Autodesk Inventor part; units mm, degrees
ref_plane "YZ Plane" through (0, 0, 0) normal (1, 0, 0) x (0, 1, 0)
ref_plane "XZ Plane" through (0, 0, 0) normal (0, 1, 0) x (-1, 0, 0)
ref_plane "XY Plane" through (0, 0, 0) normal (0, 0, 1) x (1, 0, 0)
sketch "Sketch1" plane through (0, 0, 0) normal (0, 1, 0) x (-1, 0, 0)
  circle A0 centre (0, 0) radius 5
  line L0 (0, 0) -> (12.5, 0)
  line L1 (12.5, 10) -> (12.5, -10) construction
  line L2 (11, 10) -> (11, -10)
  line L3 (14, -10) -> (14, 10)
  arc A1 (14, 10) -> (11, 10) centre (12.5, 10) ccw
  arc A2 (11, -10) -> (14, -10) centre (12.5, -10) ccw
  circle A3 centre (0, 0) radius 24
  line L4 (0, 0) -> (-33.5, 0)
  line L5 (0, 0) -> (0, 43.5)
  line L6 (-33.5, 0) -> (-33.5, 40)
  line L7 (-33.5, 40) -> (26.5, 40)
  line L8 (26.5, 40) -> (26.5, -35)
  line L9 (26.5, -35) -> (-33.5, -35)
  line L10 (-33.5, -35) -> (-33.5, 0)
  line L11 (-33.5, 40) -> (-13.5, 40)
  line L12 (-13.5, 40) -> (6.5, 40)
  line L13 (6.5, 40) -> (6.5, 45)
  line L14 (6.5, 45) -> (-13.5, 45)
  line L15 (-13.5, 45) -> (-13.5, 40)
  line L16 (-33.5, 40) -> (-33.5, 15)
  line L17 (-33.5, 15) -> (-38.5, 15)
  line L18 (-38.5, 15) -> (-38.5, -5.425)
  line L19 (-38.5, -5.425) -> (-33.5, -5.425)
  line L20 (-33.5, -5.425) -> (-33.5, 15)
  line L21 (-33.5, 15) -> (-35, 15)
  line L22 (-35, 15) -> (-35, 10)
  line L23 (-35, 10) -> (-36.5, 10)
  line L24 (-36.5, 10) -> (-36.5, 0)
  line L25 (-36.5, 0) -> (-35, 0)
  line L26 (-35, 0) -> (-35, 10)
  line L27 (6.5, 40) -> (1.5, 40)
  line L28 (1.5, 40) -> (1.5, 41.5)
  line L29 (1.5, 41.5) -> (-8.5, 41.5)
  line L30 (-8.5, 41.5) -> (-8.5, 43)
  line L31 (-8.5, 43) -> (1.5, 43)
  line L32 (1.5, 43) -> (1.5, 41.5)
  line L33 (0, 0) -> (23.3345, -23.3345)
  line L34 (0, 0) -> (33, 0) construction
  circle A4 centre (23.3345, -23.3345) radius 1.5
  circle A5 centre (23.3345, 23.3345) radius 1.5
  circle A6 centre (-23.3345, 23.3345) radius 1.5
  circle A7 centre (-23.3345, -23.3345) radius 1.5
  line L35 (-11, 10) -> (-11, -10)
  line L36 (-14, -10) -> (-14, 10)
  arc A8 (-11, 10) -> (-14, 10) centre (-12.5, 10) ccw
  arc A9 (-14, -10) -> (-11, -10) centre (-12.5, -10) ccw
  point P0 (6.5, 40)
  dimension "d0" = 10
  dimension "d1" = 12.5
  dimension "d2" = 10
  dimension "d3" = 3
  dimension "d6" = 48
  dimension "d7" = 33.5
  dimension "d8" = 43.5
  dimension "d9" = 60
  dimension "d10" = 75
  dimension "d11" = 20
  dimension "d12" = 20
  dimension "d13" = 5
  dimension "d14" = 25
  dimension "d15" = 5
  dimension "d16" = 1.5
  dimension "d17" = 5
  dimension "d18" = 1.5
  dimension "d19" = 10
  dimension "d20" = 5
  dimension "d21" = 1.5
  dimension "d22" = 10
  dimension "d23" = 1.5
  dimension "d24" = 33
  dimension "d25" = 45
  dimension "d26" = 3
  dimension "d29" = 360
extrude "Extrusion1" add sketch "Sketch1" along normal blind 2 contours A0 L5 A3 L33 | A0 L4 L35 A8 L36 A3 L5 | L33 A3 L4 L36 A9 L35 A0 | L5 L7 L8 L9 L10 L4 A3 | A3 L4 L6 L7 L5 | L7 L15 L14 L13 L28 L32 L31 L30 L29 L5 | L5 L29 L28 L7 | L26 L25 L24 L23 | L10 L19 L18 L17 L6
extrude "Extrusion2" cut sketch "Sketch1" along normal blind 2 contours L26 L25 L24 L23
sketch "Sketch2" plane through (0, 2, 0) normal (0, 1, 0) x (1, 0, 0)
  line L0 (0, -7) -> (0, 7) construction
  line L1 (5, -7) -> (5, 7)
  line L2 (-5, 7) -> (-5, -7)
  arc A0 (-5, -7) -> (5, -7) centre (0, -7) ccw
  arc A1 (5, 7) -> (-5, 7) centre (0, 7) ccw
  point P0 (0, 0)
  dimension "d35" = 7
  dimension "d36" = 10
extrude "Extrusion3" cut sketch "Sketch2" against normal blind 10
properties part number "mount"
Model file for the job. Use its own axes, mm. A direction names the side the tool comes from. Give positions to 0.01 mm unless a question says otherwise; leave off trailing zeros. Order: outer loops, then holes, each group sorted by start corner. A loop starts at its lowest first (then second) coordinate and runs counter-clockwise, first axis right, second up. Notation, with made-up numbers: (69, -34) -> (128, -34) arc R15 cw to (128, -11) -> close; hole circle Ø10 at (73, 62). An arc over 180 degrees is marked (long way). Use CSV: the item, a comma, the result in double quotes.
1. Drill centre lines: line 1 along X through (y, z) = (1.45, -7); line 2 along X through (y, z) = (1.6, 7); line 3 along Z through (x, y) = (6.5, 1.95). Where is each one in solid material? Low to high. Write a range as from..to.
Outcome:
line 1,"-26.5..-14, -11..-5, 5..11, 14..33.5"
line 2,"-26.5..-14, -11..-5, 5..11, 14..35, 36.5..38.5"
line 3,"-35..41.5, 43..45"
2. Band-saw the part on A-A, the plane z = 3. Give the cut face in (x, y), then the cut area to 3 significant figures.
Outcome:
outline,"(-26.5, 0) -> (-14, 0) -> (-14, 2) -> (-26.5, 2) -> close; (-11, 0) -> (-5, 0) -> (-5, 2) -> (-11, 2) -> close; (5, 0) -> (11, 0) -> (11, 2) -> (5, 2) -> close; (14, 0) -> (35, 0) -> (35, 2) -> (14, 2) -> close; (36.5, 0) -> (38.5, 0) -> (38.5, 2) -> (36.5, 2) -> close"
area,"95.0 mm²"
3. 3-axis set-ups, long thin cutter, end or side, ignore diameter. For faces 5 (the flat face through (-6.5, 1, 42)), 6 (the flat face through (4, 1, 43)), 7 (the flat face through (13.5, 1, 43)), 8 (the flat face through (36, 1, -5.425)): which of +Z, -Z, +X, -X, +Y, -Y reach the whole face in a straight line?
Outcome:
face 5,"+Z, -X, +Y, -Y"
face 6,"+Y, -Y"
face 7,"+Z, +X, +Y, -Y"
face 8,"-Z, +X, +Y, -Y"
4. Band-saw the part on D-D, the plane y = 1.6. Count the separate pieces of the cut face and the enclosed holes in it, then the cut area to 3 significant figures.
Outcome:
separate pieces,"1"
enclosed holes,"9"
area,"4,290 mm²"
5. Drop flat-ended pins along their axis: pin 1 (1.2 mm diameter, centred on y = 1.5, z = 42, fed in from -X); pin 2 (2.5 mm diameter, centred on x = 23.33, z = -23.33, fed in from +Y); pin 3 (1.2 mm diameter, centred on y = 1, z = 42.5, fed in from +X); pin 4 (1 mm diameter, centred on y = 1.5, z = 35.5, fed in from +X). Give the stop position or say it passes through.
Outcome:
pin 1,"x = -6.5"
pin 2,"through"
pin 3,"x = 13.5"
pin 4,"x = 33.5"
6. Band-saw the part on B-B, the plane x = 12.5. Give the cut face in (y, z).
Outcome:
outline,"(0, -35) -> (2, -35) -> (2, -11.5) -> (0, -11.5) -> close; (0, 11.5) -> (2, 11.5) -> (2, 45) -> (0, 45) -> close"
7. Band-saw the part on C-C, the plane x = 0. Give the cut face in (y, z), then the cut area to 3 significant figures.
Outcome:
outline,"(0, -35) -> (2, -35) -> (2, -12) -> (0, -12) -> close; (0, 12) -> (2, 12) -> (2, 41.5) -> (0, 41.5) -> close; (0, 43) -> (2, 43) -> (2, 45) -> (0, 45) -> close"
area,"109 mm²"
8. Mould opens along Z. For faces 1 (the flat face through (24, 1, 40)), 2 (the cylindrical face through (23.66, 0.99, -21.87)), 3 (the flat face through (3, 1, -35)), 4 (the flat face through (6, 0, 6)) say: +Z half, -Z half, draft (parallel to the pull), parting line (faces both ways), or undercut.
Outcome:
face 1,"+Z half"
face 2,"undercut"
face 3,"-Z half"
face 4,"draft"
